Can you work these out from the model? Positions are in its coordinate system, mm. Face numbers are marked on the shaded views. A direction names the side the tool comes from. Give positions to 0.01 mm unless a question says otherwise; leave off trailing zeros. Loops run counter-clockwise (first coordinate to the right, second up) from the corner with the lowest first, then second, coordinate; pieces in that order, holes last. Notation, with made-up numbers: (-4.75, -9) -> (11.25, -9) arc R14 ccw to (11.25, 14) -> close; hole circle Ø8 at (82, -8). An arc over 180 degrees is marked (long way). Use CSV: the item, a comma, the result in double quotes.
Autodesk Inventor part; units mm, degrees
ref_plane "YZ Plane" through (0, 0, 0) normal (1, 0, 0) x (0, 1, 0)
ref_plane "XZ Plane" through (0, 0, 0) normal (0, 1, 0) x (-1, 0, 0)
ref_plane "XY Plane" through (0, 0, 0) normal (0, 0, 1) x (1, 0, 0)
sketch "Sketch1" plane through (0, 0, 0) normal (0, 0, 1) x (1, 0, 0)
  line L0 (0, 0) -> (0, 15)
  line L1 (0, 15) -> (2, 15)
  line L2 (0, 0) -> (6, 0)
  line L3 (6, 0) -> (6, 11)
  line L4 (6, 11) -> (2, 15)
  dimension "d0" = 15
  dimension "d1" = 2
  dimension "d2" = 6
  dimension "d3" = 11
extrude "Extrusion1" add sketch "Sketch1" along normal blind 10
sketch "Sketch2" plane through (0, 0, 0) normal (0, 0, -1) x (-1, 0, 0)
  line L0 (0, 15) -> (0, 0)
  line L1 (0, 0) -> (-3, 0)
  line L2 (0, 0) -> (-6, 0)
  line L3 (-6, 11) -> (-2, 15)
  line L4 (0, 0) -> (3, 0)
  line L5 (0, 11) -> (-3, 8)
  line L6 (0, 11) -> (3, 8)
  line L7 (-3, 8) -> (-3, 0)
  line L8 (3, 8) -> (3, 0)
extrude "Extrusion2" add sketch "Sketch2" along normal blind 28
sketch "Sketch3" plane through (0, 0, -28) normal (0, 0, -1) x (-1, 0, 0)
  line L0 (0, 15) -> (0, 0)
  line L1 (0, 0) -> (-6, 0)
  line L2 (0, 0) -> (-6, 0)
  line L3 (-6, 0) -> (-6, 11)
  line L4 (-6, 0) -> (-6, 11)
  line L5 (-6, 11) -> (-2, 15)
  line L6 (-6, 11) -> (-2, 15)
  line L7 (-2, 15) -> (0, 15)
  line L8 (-2, 15) -> (0, 15)
  line L9 (0, 15) -> (0, 0)
extrude "Extrusion3" add sketch "Sketch3" along normal blind 10
properties part number "inside-join"
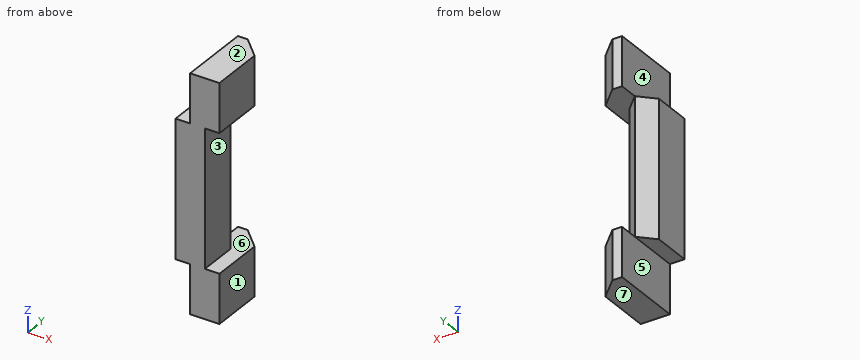
(1) Will these pins go through, and if not, where does the flat tip stop? pin 1 Ø1 at (x, z) = (-2, -1) entering from +Y; pin 2 Ø1.5 at (x, z) = (-1, -28.5) entering from +Y; pin 3 Ø1.5 at (x, y) = (-1, 9.5) entering from +Z.
Answer sheet:
pin 1,"stops at y = 9.5"
pin 2,"stops at y = 10.56"
pin 3,"stops at z = 0"
(2) We'd pull the mould along Z, two halves only. Please class the marked faces 1, 2 and 3: released by +Z, released by -Z, zero draft, split by the parting line, or undercut.
Answer sheet:
face 1,"zero draft"
face 2,"released by +Z"
face 3,"undercut"
(3) If we section it at A-A, the plane x = 4.5: Write out the boundary of the cut face in (y, z).
Answer sheet:
outline,"(0, -38) -> (12.5, -38) -> (12.5, -28) -> (0, -28) -> close; (0, 0) -> (12.5, 0) -> (12.5, 10) -> (0, 10) -> close"
(4) If we section it at C-C, the plane y = 12.5: Write out the boundary of the cut face in (x, z).
Answer sheet:
outline,"(0, -38) -> (4.5, -38) -> (4.5, -28) -> (0, -28) -> close; (0, 0) -> (4.5, 0) -> (4.5, 10) -> (0, 10) -> close"
(5) If we section it at B-B, the plane y = 8.75: Write out the boundary of the cut face in (x, z).
Answer sheet:
outline,"(-2.25, -28) -> (0, -28) -> (0, -38) -> (6, -38) -> (6, -28) -> (2.25, -28) -> (2.25, 0) -> (6, 0) -> (6, 10) -> (0, 10) -> (0, 0) -> (-2.25, 0) -> close"
(6) Which directions (+Z, -Z, +X, -X, +Y, -Y) give clear straight access to the entire face, cutting with the end or side of a thin tool? Please do the marked faces 4, 5, 6 and 7.
Answer sheet:
face 4,"+Z, -X, +Y, -Y"
face 5,"-Z, -X, +Y, -Y"
face 6,"+X, +Y"
face 7,"-Z, +X, -X, +Y, -Y"
(7) If we section it at D-D, the plane z = 1: Write out the boundary of the cut face in (x, y), then the cut area to 3 significant figures.
Answer sheet:
outline,"(0, 0) -> (6, 0) -> (6, 11) -> (2, 15) -> (0, 15) -> close"
area,"82.0 mm2"
(8) If I drill on L1, parallel to Z at x = 0.5, y = 13; L2, parallel to X at y = 10.5, z = 3; L3, parallel to Z at x = -2, y = 5.5, over which ranges is the centre line in solid material (lowest first)? Write a range as from..to.
Answer sheet:
L1,"z = -38..-28, 0..10"
L2,"x = 0..6"
L3,"z = -28..0"
